Answer from the drawing. Dimensions are ordinates in mm from the lowest x, y and z of the part. A direction names the side the tool comes from. Give positions to 0.01 mm unless a question says otherwise; leave off trailing zeros. Loops run counter-clockwise (first coordinate to the right, second up) from the corner with the lowest first, then second, coordinate; pieces in that order, holes last.
Item 1: Section C-C, the plane z = 35.5 is taken. Give the vertices of the cut face in (x, y).
Item 2: Section D-D, the plane z = 27.5 is taken. Give the vertices of the cut face in (x, y).
Item 3: A tool of negligible diameter and unlimited length cuts with its end or side. For the marked faces 4 and 5, from which of +Z, -Z, +X, -X, +Y, -Y can it reach the whole face along a straight path? Write none if from no direction.
Item 4: Each of these flat-tipped pins is pushed along its axis until it touches: pin 1 Ø12 at (x, z) = (107, 27) entering from +Y; pin 2 Ø1.5 at (y, z) = (107.5, 21) entering from +X; pin 3 Ø6 at (x, z) = (53.5, 25.5) entering from -Y. Where does it stop, or does it pass through?
Item 5: The mould has two halves that part along Y. Classify the marked faces 1, 2 and 3: pulls with the +Y half, pulls with the -Y half, needs draft (parallel to the pull), parting line crosses it, or undercut.
Item 6: Section A-A, the plane y = 63.5 is taken. Give the vertices of the cut face in (x, z).
Item 7: Consider line 1 along Y through (x, z) = (63.5, 35.35); line 2 along X through (y, z) = (63, 34); line 3 along Y through (x, z) = (63, 14). Determine where each line is inside the solid, lowest interval first.
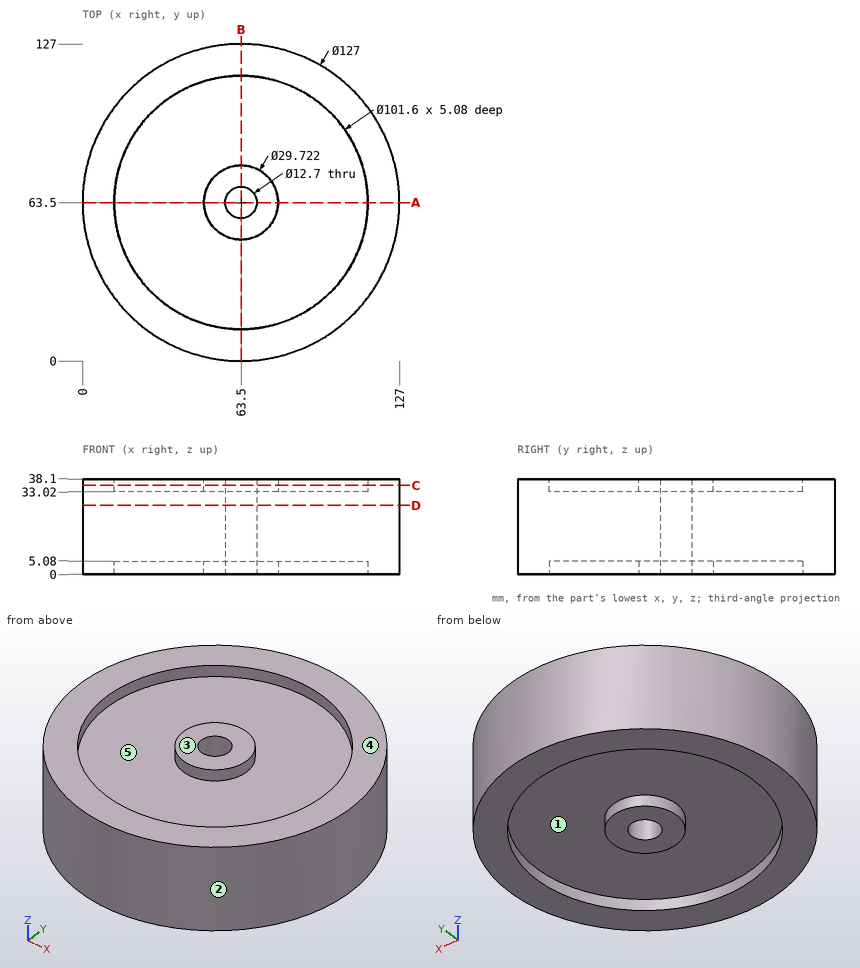
Worked answers:
1. outline: circle Ø127 at (63.5, 63.5); circle Ø29.72 at (63.5, 63.5); hole circle Ø101.6 at (63.5, 63.5); hole circle Ø12.7 at (63.5, 63.5)
2. outline: circle Ø127 at (63.5, 63.5); hole circle Ø12.7 at (63.5, 63.5)
3. face 4: +Z, +X, -X, +Y, -Y
3. face 5: +Z
4. pin 1: stops at y = 114.74
4. pin 2: stops at x = 109.99
4. pin 3: stops at y = 0.39
5. face 1: undercut
5. face 2: parting line crosses it
5. face 3: needs draft
6. outline: (0, 0) - (12.7, 0) - (12.7, 5.08) - (48.64, 5.08) - (48.64, 0) - (57.15, 0) - (57.15, 38.1) - (48.64, 38.1) - (48.64, 33.02) - (12.7, 33.02) - (12.7, 38.1) - (0, 38.1) - close; (69.85, 0) - (78.36, 0) - (78.36, 5.08) - (114.3, 5.08) - (114.3, 0) - (127, 0) - (127, 38.1) - (114.3, 38.1) - (114.3, 33.02) - (78.36, 33.02) - (78.36, 38.1) - (69.85, 38.1) - close
7. line 1: y = 0 to 12.7, 48.64 to 57.15, 69.85 to 78.36, 114.3 to 127
7. line 2: x = 0 to 12.7, 48.65 to 57.17, 69.83 to 78.35, 114.3 to 127
7. line 3: y = 0 to 57.17, 69.83 to 127
